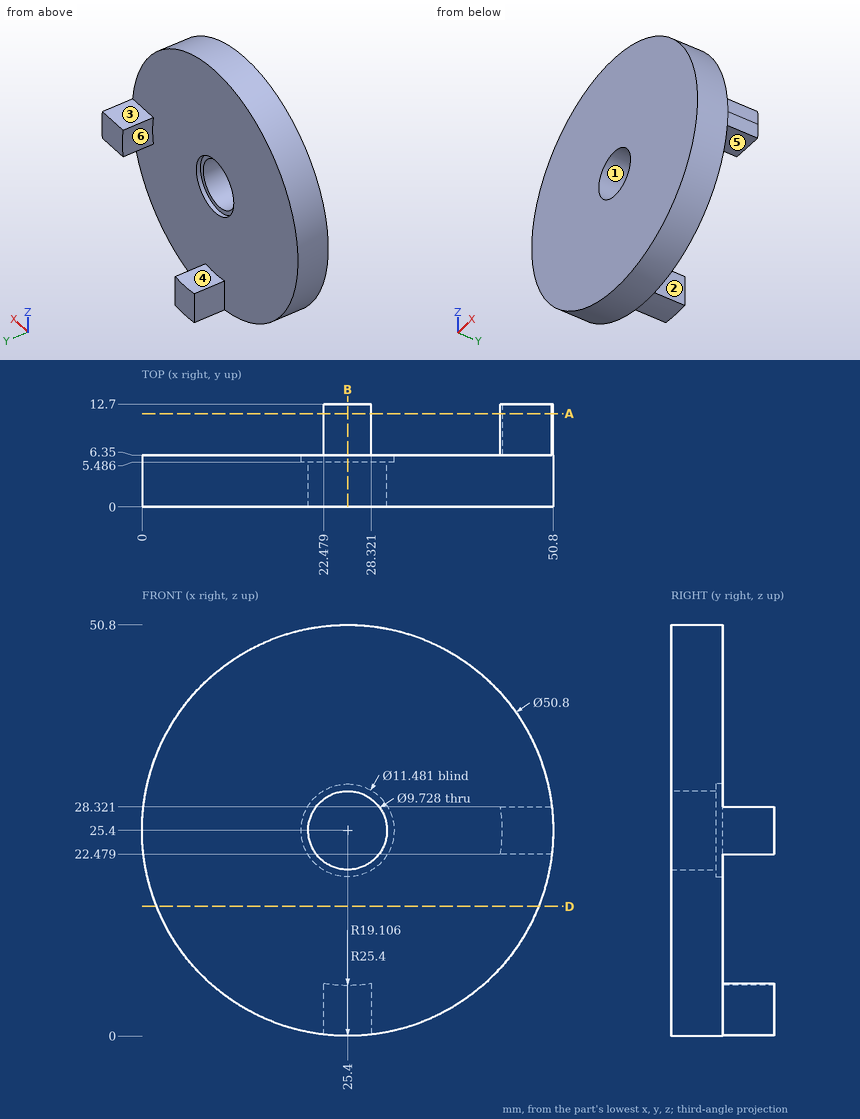
The drawing under review shows one solid part. Ordinate dimensions are in mm from its lowest x, y, z. A direction names the side the tool comes from. Round coordinates to 2 decimals unless told otherwise and drop trailing zeros. Loops run counter-clockwise (first coordinate to the right, second up) from the corner with the lowest first, then second, coordinate; pieces in that order, holes last. Notation, with made-up numbers: (70.25, 24) - (85.25, 24) arc R30 cw to (85.25, 55) - close; hole circle Ø6 at (-8, 64). An arc over 180 degrees is marked (long way). One line per item, written item: value. Start each with the question number.
1) Consider section B-B on x = 25.4. Give the boundary of the cut face in (y, z), then the cut area to 3 significant figures.
2) To check wall thickness, follow L1, parallel to X at y = 6.05, z = 25.4; L2, parallel to X at y = 2.15, z = 25.4; L3, parallel to Y at x = 33, z = 40.5. State the ranges of each line that lie inside material, in increasing order. Write a range as from..to.
3) Draft analysis for pull direction X (two halves, no side actions). For the marked faces 1, 2 and 3, state which applies: +X half, -X half, draft (parallel to the pull), parting line (faces both ways), or undercut.
4) Consider section D-D on z = 16. Give the boundary of the cut face in (x, y).
5) For the marked faces 4, 5 and 6, list the 3-axis set-ups (+Z, -Z, +X, -X, +Y, -Y) from which the entire face can be reached by the end or side of a thin tool; tool diameter is ignored.
6) Consider section A-A on y = 11.5. Give the boundary of the cut face in (x, z).
7) Insertion check: pin 1 Ø6 at (x, z) = (39, 33) entering from +Y; pin 2 Ø5 at (y, z) = (11, 4) entering from +X; pin 3 Ø10 at (x, z) = (25.5, 7) entering from -Y; pin 4 Ø4 at (x, y) = (14, 3.5) entering from -Z. Each pin has a flat end and moves straight along its axis. Give the tip position at first contact, or say it passes through.
Reported:
1. outline: (0, 0) - (12.7, 0) - (12.7, 6.29) - (6.35, 6.29) - (6.35, 19.66) - (5.49, 19.66) - (5.49, 20.54) - (0, 20.54) - close; (0, 30.26) - (5.49, 30.26) - (5.49, 31.14) - (6.35, 31.14) - (6.35, 50.8) - (0, 50.8) - close
1. area: 299 mm^2
2. L1: x = 0..19.66, 31.14..50.8
2. L2: x = 0..20.54, 30.26..50.8
2. L3: y = 0..6.35
3. face 1: undercut
3. face 2: +X half
3. face 3: draft
4. outline: (1.8, 0) - (49, 0) - (49, 6.35) - (1.8, 6.35) - close
5. face 4: +Z, +Y
5. face 5: -Z, +X, -X, +Y
5. face 6: -X, +Y
6. outline: (22.48, 0.17) arc R25.4 ccw to (28.32, 0.17) - (28.32, 6.52) arc R19.11 cw to (22.48, 6.52) - close; (44.28, 22.48) - (50.63, 22.48) arc R25.4 ccw to (50.63, 28.32) - (44.28, 28.32) arc R19.11 cw to start
7. pin 1: stops at y = 6.35
7. pin 2: stops at x = 28.32
7. pin 3: stops at y = 0
7. pin 4: stops at z = 1.8
